from build123d import *

# Parameters (mm, degrees)
EXTRUDE_1_DEPTH     = 144.8
SKETCH_7_R          = 1.5
CUT_EXTRUDE_6_DEPTH = 80
CUT_EXTRUDE_START   = -125
CUT_EXTRUDE_8_DEPTH = 125


with BuildPart() as part:
    # 草图1 → 凸台-拉伸1 (new body)
    with BuildSketch(Plane.XY):
        with BuildLine():
            Line((-55, 0), (-51.8, 0))
            ThreePointArc((-51.8, 0), (-17.476086779, -48.76296126), (40.00796876, -32.902924425))
            ThreePointArc((40.00796876, -32.902924425), (41.062164054, -31.150956215), (41.565129022, -29.16910189))
            Line((41.565129022, -29.16910189), (41.910264928, -25.795992674))
            ThreePointArc((41.910264928, -25.795992674), (42.185460224, -24.44340265), (42.720717667, -23.171108779))
            ThreePointArc((42.720717667, -23.171108779), (47.564735827, -9.977770578), (48.43095601, 4.05))
            ThreePointArc((48.43095601, 4.05), (47.472400425, 6.007940217), (45.441390824, 6.8))
            Line((45.441390824, 6.8), (31, 6.8))
            ThreePointArc((31, 6.8), (30.292893219, 7.092893219), (30, 7.8))
            Line((30, 7.8), (30, 9))
            ThreePointArc((30, 9), (30.292893219, 9.707106781), (31, 10))
            Line((31, 10), (50.344019583, 10))
            ThreePointArc((50.344019583, 10), (50.805346897, 9.459374484), (51.0484918, 8.791557597))
            ThreePointArc((51.0484918, 8.791557597), (51.611780996, 4.411809423), (51.8, 0))
            Line((51.8, 0), (55, 0))
            ThreePointArc((55, 0), (0, -55), (-55, 0))
        make_face()
    extrude(amount=EXTRUDE_1_DEPTH)

    # 草图7 → 切除-拉伸6 (cut)
    with BuildSketch(Plane(origin=(0, 0, 0), x_dir=(0.10066073352284005, 0.994920809274107, 0), z_dir=(-0.9949208092741069, 0.10066073352284004, 0))):
        with Locations(Location((-0.136340344, -18.9, 0), (0, 0, 180))):
            Circle(SKETCH_7_R)
        with Locations(Location((-0.136340344, -38.9, 0), (0, 0, 180))):
            Circle(SKETCH_7_R)
        with Locations(Location((-0.136340344, -105.9, 0), (0, 0, 180))):
            Circle(SKETCH_7_R)
        with Locations(Location((-0.136340344, -125.9, 0), (0, 0, 180))):
            Circle(SKETCH_7_R)
    extrude(amount=-CUT_EXTRUDE_6_DEPTH, mode=Mode.SUBTRACT)

    # 草图4 → 切除-拉伸8 (cut)
    with BuildSketch(Plane.XY.offset(144.8).offset(CUT_EXTRUDE_START)):
        with BuildLine():
            Line((55, 0), (0, 0))
            Line((0, 0), (50.016978469, 22.875792113))
            ThreePointArc((50.016978469, 22.875792113), (53.739807479, 11.70611345), (55, 0))
        make_face()
    extrude(amount=CUT_EXTRUDE_8_DEPTH, mode=Mode.SUBTRACT)


solid = part.part
For this review, take the finished solid that the model builds, in its own axes (mm). A direction names the side the tool comes from. Give positions to 0.01 mm unless a question says otherwise; leave off trailing zeros. Order: outer loops, then holes, each group sorted by start corner. A loop starts at its lowest first (then second) coordinate and runs counter-clockwise, first axis right, second up. Notation, with made-up numbers: M 10.5,19 L 17.5,19 A27 cw 17.5,47 Z; hole C 36,36.25 d2. An arc over 180 degrees is marked long. Answer in a Markdown table with one row per item. Add a question column.
(1) For faces 5 (the face through (25, -46, 0)), 6 (the face through (38, 6.8, 10)), 7 (the face through (43, 7, 19.8)), 8 (the face through (47.524, -10.171, 71.386)), list the 3-axis set-ups (+Z, -Z, +X, -X, +Y, -Y) from which the entire face can be reached by the end or side of a thin tool; tool diameter is ignored.
(2) Consider section B-B on x = 34.5. State the section outline as (y, z) points, and give its area (3 significant figures).
(3) Wall thickness on probe 1 along X at (y, z) = (-1.5, 98); probe 2 along X at (y, z) = (-43, 74); probe 3 along Y at (x, z) = (6, 96): over which ranges is each line inside the solid? List them lowest first. Write a range as [from, to].
(4) Mouldability with a two-part tool opening along X and no side actions: class faces 1 (the face through (-53, 0, 71)), 2 (the face through (51.585, -4.16, 37.987)), 3 (the face through (51.606, 4.473, 9.761)), 4 (the face through (51.395, -6.033, 104.569)) as +X half, -X half, draft (parallel to the pull), parting line (faces both ways), or undercut.
(5) Consider section D-D on z = 70. State the section outline as (x, y) points.
(6) Consider section C-C on x = 0. State the section outline as (y, z) points, and give its area (3 significant figures).
(7) Consider section A-A on z = 11. State the section outline as (x, y) points, and give its area (3 significant figures).
(8) For pin 1 (10 mm diameter, centred on y = -27.5, z = 20.5, fed in from +X); pin 2 (1 mm diameter, centred on x = -53, z = 55, fed in from +Y); pin 3 (0.6 mm diameter, centred on y = 8, z = 10, fed in from -X), all flat-tipped, find the tip position at first contact; note any pin that passes through.
Evaluation:
| question | item | result |
|---|---|---|
| 1 | face 5 | -Z, +X, -X, +Y, -Y |
| 1 | face 6 | +Z, -Z, -X |
| 1 | face 7 | +Z, +X, -X, +Y |
| 1 | face 8 | +Z, -Z |
| 2 | outline | M -42.83,0 L -38.64,0 L -38.64,144.8 L -42.83,144.8 Z; M 6.8,0 L 10,0 L 10,19.8 L 6.8,19.8 Z |
| 2 | area | 671 mm^2 |
| 3 | probe 1 | x = [-54.98, -51.78], [48.58, 54.98] |
| 3 | probe 2 | x = [-34.29, -28.88], [28.88, 34.29] |
| 3 | probe 3 | y = [-54.67, -51.45] |
| 4 | face 1 | draft |
| 4 | face 2 | undercut |
| 4 | face 3 | +X half |
| 4 | face 4 | undercut |
| 5 | outline | M -55,0 A55 ccw 55,0 L 48.6,0 A48.6 cw 42.72,-23.17 A7 ccw 41.91,-25.8 L 41.57,-29.17 A7 cw 40.01,-32.9 A51.8 cw -51.8,0 Z |
| 6 | outline | M -55,0 L -51.8,0 L -51.8,144.8 L -55,144.8 Z |
| 6 | area | 463 mm^2 |
| 7 | outline | M -55,0 A55 ccw 55,0 L 51.8,0 A51.8 ccw 51.05,8.79 A2 ccw 50.34,10 L 31,10 A1 ccw 30,9 L 30,7.8 A1 ccw 31,6.8 L 45.44,6.8 A3 cw 48.43,4.05 A48.6 cw 42.72,-23.17 A7 ccw 41.91,-25.8 L 41.57,-29.17 A7 cw 40.01,-32.9 A51.8 cw -51.8,0 Z |
| 7 | area | 722 mm^2 |
| 8 | pin 1 | stops at x = 50.19 |
| 8 | pin 2 | stops at y = 0 |
| 8 | pin 3 | stops at x = 30 |
